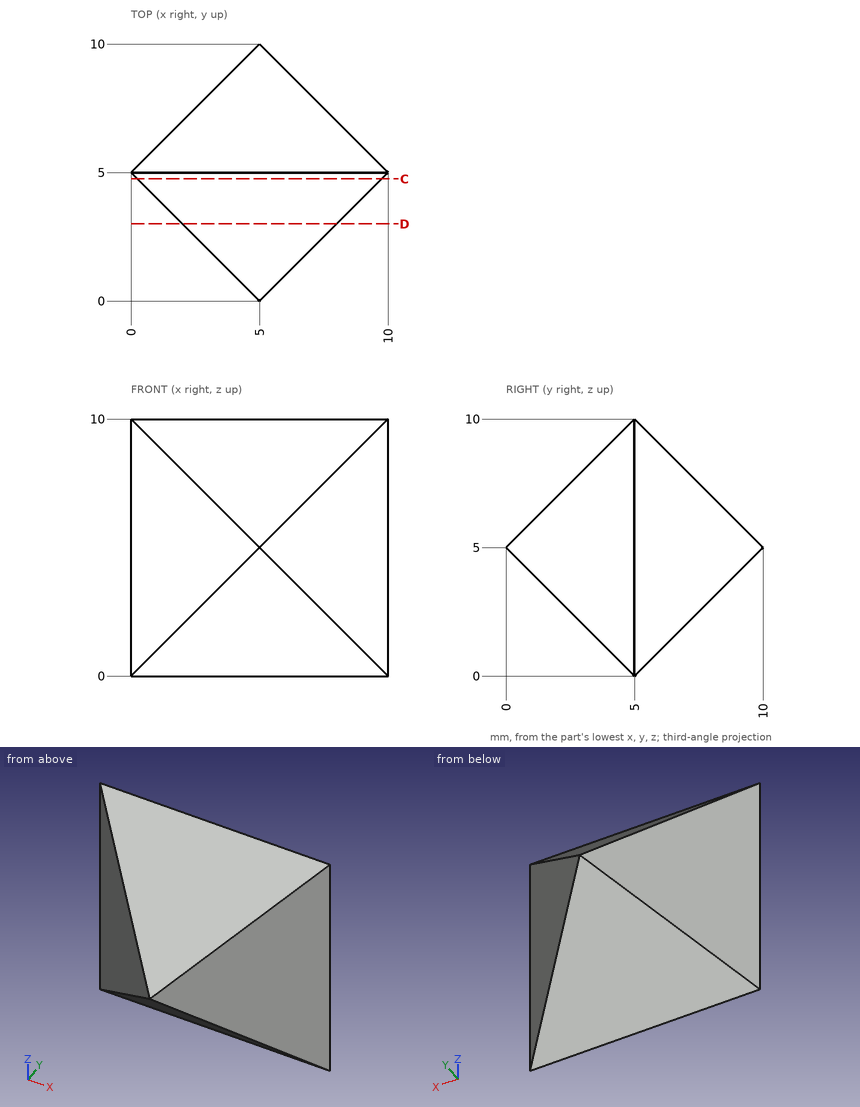
For this review, use the dimensioned drawing (mm, ordinates from the lowest corner) and the shaded views. Give positions to 0.01 mm unless a question says otherwise; leave off trailing zeros. Write each loop counter-clockwise with the first axis right and the second up, starting at its lowest first coordinate (ties: lowest second). Pieces come first, ordered by that corner, then holes.
(1) For P1, Ø1.5, axis at x = 7.5, y = 2.5, coming from the +Z side; P2, Ø2, axis at x = 5, y = 1, coming from the -Z side; P3, Ø6, axis at x = 1, z = 2.5, coming from the -Y side, all flat-tipped, find the tip position at first contact; note any pin that passes through.
(2) Consider section C-C, the plane y = 4.75. Give the boundary of the cut face in (x, z), and give its area (4 significant figures).
(3) To check wall thickness, follow L1, parallel to X at y = 7, z = 5.75; L2, parallel to Z at x = 4.25, y = 6.5; L3, parallel to Y at x = 9.25, z = 8.25. State the ranges of each line that lie inside material, in increasing order.
(4) Consider section D-D, the plane y = 3. Give the boundary of the cut face in (x, z).
Returned:
1. P1: stops at z = 8.25
1. P2: stops at z = 3
1. P3: stops at y = 1.27
2. outline: (0.25, 0.25) - (9.75, 0.25) - (9.75, 9.75) - (0.25, 9.75) - close
2. area: 90.25 mm2
3. L1: x = 2 to 8
3. L2: z = 1.5 to 8.5
3. L3: y = 4.25 to 5.75
4. outline: (2, 2) - (8, 2) - (8, 8) - (2, 8) - close
